Can you work these out from the model? Positions are in its coordinate system, mm. A direction names the side the tool comes from. Round coordinates to 2 decimals unless told otherwise and drop trailing zeros. Loops run counter-clockwise (first coordinate to the right, second up) from the corner with the lowest first, then second, coordinate; pieces in that order, holes last. Notation, with made-up numbers: (24.5, -34) -> (68.5, -34) arc R22 ccw to (68.5, -9) -> close; hole circle Ø5 at (89, 69.5). An arc over 180 degrees is marked (long way). Write each question's results on one line, items separated by ' | '.
from build123d import *

# Parameters (mm, degrees)
SKETCH_1_R          = 8
EXTRUDE_1_DEPTH     = 23
SKETCH_2_R          = 6
EXTRUDE_2_DEPTH     = 27
SKETCH_3_R          = 1.5
EXTRUDE_3_DEPTH     = 12
SKETCH_4_R          = 2
EXTRUDE_4_DEPTH     = 2
SKETCH_5_R          = 7.5
EXTRUDE_6_DEPTH     = 25
CUT_EXTRUDE_2_DEPTH = 25
SKETCH_7_W          = 0.238746812
SKETCH_7_H          = 2.029347906
SKETCH_7_W_2        = 0.208903461
EXTRUDE_7_DEPTH     = 4
SKETCH_8_R          = 0.451828616
CUT_EXTRUDE_3_DEPTH = 40
SKETCH_9_W          = 4.595876138
SKETCH_9_H          = 0.537180328
CUT_EXTRUDE_4_DEPTH = 6


with BuildPart() as part:
    # 草图1 → 凸台-拉伸1 (new body)
    with BuildSketch(Plane.XY):
        Circle(SKETCH_1_R)
    extrude(amount=EXTRUDE_1_DEPTH)

    # 草图2 → 凸台-拉伸2 (add)
    with BuildSketch(Plane(origin=(0, 0, 0), x_dir=(-1, 0, 0), z_dir=(0, 0, -1))):
        Circle(SKETCH_2_R)
    extrude(amount=EXTRUDE_2_DEPTH)

    # 草图3 → 凸台-拉伸3 (add)
    with BuildSketch(Plane.XY.offset(23)):
        Circle(SKETCH_3_R)
    extrude(amount=EXTRUDE_3_DEPTH)

    # 草图4 → 凸台-拉伸4 (add)
    with BuildSketch(Plane.XY.offset(23)):
        Circle(SKETCH_4_R)
    extrude(amount=EXTRUDE_4_DEPTH)

    # 草图5 → 凸台-拉伸6 (add)
    with BuildSketch(Plane(origin=(0, 0, 0), x_dir=(-1, 0, 0), z_dir=(0, 0, -1))):
        with Locations(Location((0, 0, 0), (0, 0, 180))):
            Circle(SKETCH_5_R)
    extrude(amount=EXTRUDE_6_DEPTH)

    # 草图6 → 切除-拉伸2 (cut)
    with BuildSketch(Plane(origin=(0, 0, -25), x_dir=(-1, 0, 0), z_dir=(0, 0, -1))):
        Polygon((0, -6), (7.251934426, -6), (7.251934426, -9), (-7.072874317, -9), (-7.072874317, -6), align=None)
    extrude(amount=-CUT_EXTRUDE_2_DEPTH, mode=Mode.SUBTRACT)

    # 草图7 → 凸台-拉伸7 (add)
    with BuildSketch(Plane(origin=(0, 0, -27), x_dir=(-1, 0, 0), z_dir=(0, 0, -1))):
        with Locations((-5.40164663, 0)):
            Rectangle(SKETCH_7_W, SKETCH_7_H)
        with Locations((5.371803278, 0)):
            Rectangle(SKETCH_7_W_2, SKETCH_7_H)
    extrude(amount=EXTRUDE_7_DEPTH)

    # 草图8 → 切除-拉伸3 (cut)
    with BuildSketch(Plane(origin=(5.521020036, 0, 0), x_dir=(0, 0, -1), z_dir=(1, 0, 0))):
        with Locations((30.17785099, 0)):
            Circle(SKETCH_8_R)
    extrude(amount=-CUT_EXTRUDE_3_DEPTH, mode=Mode.SUBTRACT)

    # 草图9 → 切除-拉伸4 (cut)
    with BuildSketch(Plane.XY.offset(35)):
        with Locations((0, -1.268342441)):
            Rectangle(SKETCH_9_W, SKETCH_9_H)
    extrude(amount=-CUT_EXTRUDE_4_DEPTH, mode=Mode.SUBTRACT)


solid = part.part
1. If we section it at A-A (z = 4.5): List the corners of the cut face in (x, y) for me.
Final values:
outline: circle Ø16 at (0, 0)
2. If we section it at C-C (z = -18): List the corners of the cut face in (x, y) for me, then the cut area to 3 significant figures.
Final values:
outline: (-4.5, -6) -> (4.5, -6) arc R7.5 ccw (long way) to start | area: 168 mm2
3. Will these pins go through, and if not, where does the flat tip stop? pin 1 (1.5 mm diameter, centred on y = 3, z = 1.5, fed in from +X); pin 2 (3.5 mm diameter, centred on x = 1.5, y = 0, fed in from -Z); pin 3 (2 mm diameter, centred on y = -0.5, z = -29.5, fed in from -X).
Final values:
pin 1: x = 7.68 | pin 2: z = -27 | pin 3: x = -5.48
4. On a 3-axis mill with a long thin cutter (end or side, diameter ignored), from which of +Z, -Z, +X, -X, +Y, -Y can I reach the whole of each face in a straight line? I mean faces 1 (the face through (5.282, 0, -29)), 2 (the face through (0.5, 6.2, -25)), 3 (the face through (2, -2, 23)), 4 (the face through (0, -1, 32)). Say none if no direction works.
Final values:
face 1: -Z, +Y, -Y | face 2: -Z | face 3: +Z | face 4: +Z, +X, -X, -Y
5. Please list where these lines run through material, in increasing order: line 1 (Z direction, x = 4.5, y = 3.5); line 2 (Y direction, x = 0.25, z = 20); line 3 (Z direction, x = -5, y = 5.75). Write a range as from..to.
Final values:
line 1: -27..23 | line 2: -8..8 | line 3: 0..23
6. If we section it at B-B (y = -3.5): List the corners of the cut face in (x, z) for me, then the cut area to 3 significant figures.
Final values:
outline: (-7.19, 0) -> (-6.63, 0) -> (-6.63, -25) -> (-4.87, -25) -> (-4.87, -27) -> (4.87, -27) -> (4.87, -25) -> (6.63, -25) -> (6.63, 0) -> (7.19, 0) -> (7.19, 23) -> (-7.19, 23) -> close | area: 682 mm2
7. We'd pull the mould along X, two halves only. Please class faces 5 (the face through (6, 0, -26)), 6 (the face through (0, -6, -13)), 7 (the face through (-5.267, 0, -29)), 8 (the face through (0, 0, -27)): pulls with the +X half, pulls with the -X half, needs draft (parallel to the pull), parting line crosses it, or undercut.
Final values:
face 5: parting line crosses it | face 6: needs draft | face 7: undercut | face 8: undercut
